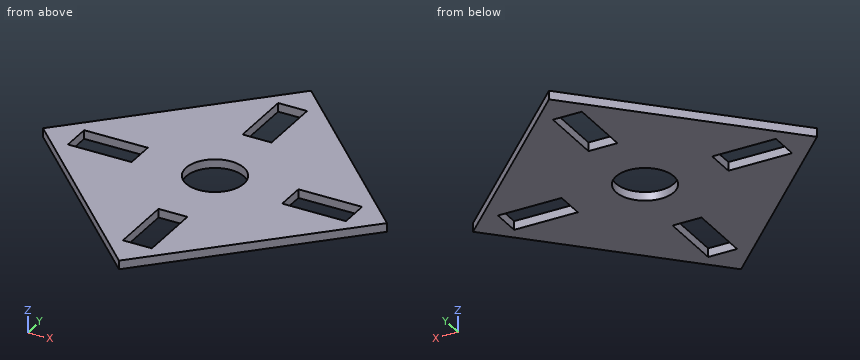
```python
from build123d import *

# Parameters (mm, degrees)
SKETCH_R   = 5
SKETCH_W   = 11
SKETCH_H   = 5
SKETCH_W_2 = 5
SKETCH_H_2 = 11
PAD_DEPTH  = 1.5


with BuildPart() as part:
    # Sketch → Pad (new body)
    with BuildSketch(Plane.XY):
        Polygon((29.698485, 0), (0, 29.698485), (-29.698485, 0), (0, -29.698485), align=None)
        Circle(SKETCH_R, mode=Mode.SUBTRACT)
        with Locations((-18.5, 0)):
            Rectangle(SKETCH_W, SKETCH_H, mode=Mode.SUBTRACT)
        with Locations((0, 18.5)):
            Rectangle(SKETCH_W_2, SKETCH_H_2, mode=Mode.SUBTRACT)
        with Locations((0, -18.5)):
            Rectangle(SKETCH_W_2, SKETCH_H_2, mode=Mode.SUBTRACT)
        with Locations((18.5, 0)):
            Rectangle(SKETCH_W, SKETCH_H, mode=Mode.SUBTRACT)
    extrude(amount=PAD_DEPTH)


solid = part.part
```
Model file for the job. Use its own axes, mm. Coordinates: 2 decimals unless noted, no trailing zeros. Loops run counter-clockwise (first coordinate to the right, second up) from the corner with the lowest first, then second, coordinate; pieces in that order, holes last. Notation, with made-up numbers: (60.5, 79.5) -> (96.5, 79.5) arc R17 ccw to (96.5, 91.5) -> close; hole circle Ø4 at (-30.5, 45). An arc over 180 degrees is marked (long way). Answer as a JSON object with one key per item and string values.
Q1. Flat gauge pins, fed straight in: P1, Ø0.8, axis at y = -20, z = 0.5, coming from the -X side; P2, Ø0.8, axis at y = 19, z = 1, coming from the +X side. Where does each tip first touch, or does it go through?
Report:
{"P1": "stops at x = -10.1", "P2": "stops at x = 11.1"}
Q2. Cut at A-A (z = 1.1). List the corners of the cut face in (x, y).
Report:
{"outline": "(-29.7, 0) -> (0, -29.7) -> (29.7, 0) -> (0, 29.7) -> close; hole (-24, -2.5) -> (-13, -2.5) -> (-13, 2.5) -> (-24, 2.5) -> close; hole circle Ø10 at (0, 0); hole (-2.5, -24) -> (2.5, -24) -> (2.5, -13) -> (-2.5, -13) -> close; hole (-2.5, 13) -> (2.5, 13) -> (2.5, 24) -> (-2.5, 24) -> close; hole (13, -2.5) -> (24, -2.5) -> (24, 2.5) -> (13, 2.5) -> close"}
Q3. Cut at B-B (x = 16). List the corners of the cut face in (y, z), and give its area (3 significant figures).
Report:
{"outline": "(-13.7, 0) -> (-2.5, 0) -> (-2.5, 1.5) -> (-13.7, 1.5) -> close; (2.5, 0) -> (13.7, 0) -> (13.7, 1.5) -> (2.5, 1.5) -> close", "area": "33.6 mm2"}
Q4. Cut at C-C (y = -19). List the corners of the cut face in (x, z).
Report:
{"outline": "(-10.7, 0) -> (-2.5, 0) -> (-2.5, 1.5) -> (-10.7, 1.5) -> close; (2.5, 0) -> (10.7, 0) -> (10.7, 1.5) -> (2.5, 1.5) -> close"}
Q5. Probe probe 1 along Y at (x, z) = (-1, 0.3); probe 2 along X at (y, z) = (4, 0.6); probe 3 along Y at (x, z) = (-13.5, 1.1). List the from-to ranges inside material, lowest first.
Report:
{"probe 1": "y = -28.7 to -24, -13 to -4.9, 4.9 to 13, 24 to 28.7", "probe 2": "x = -25.7 to -3, 3 to 25.7", "probe 3": "y = -16.2 to -2.5, 2.5 to 16.2"}
